```python
from build123d import *

# Parameters (mm, degrees)
F0_R     = 4.2534442679
F1_DEPTH = 20
F2_W     = 10.3906942531
F2_H     = 12.2660957277
F2_W_2   = 9.8304990679
F2_W_3   = 9.2522380874
F2_W_4   = 10.9689552337
F3_DEPTH = 10.16
F5_R     = 6.35
F6_DEPTH = 25.4
F7_R     = 6.35
F8_DEPTH = 25.4
F4_W     = 109.22
F4_H     = 58.420000254
F9_DEPTH = 12.7


# Not quite as in the source:
# - a feature names something its author has since deleted; it is built from what else it names


with BuildPart() as f1:
    # F0 (on Top) → F1 (new body)
    with BuildSketch(Plane.XY):
        Polygon((-67.5837442279, -21.374759078), (-67.5837442279, -75), (-7.2734476998, -75), (0, -75), (67.5837334, -75), (67.5837334, -21.374759078), (75, -21.374759078), (75, -5.6661395316), (75, 75), (-75, 75), (-75, -5.6661395316), (-75, -21.374759078), align=None)
        with BuildLine():
            ThreePointArc((-190.7009859405, 27.2364963511), (-152.5558792144, -43.9704630954), (-75, -21.374759078))
            Line((-75, -21.374759078), (-75, -5.6661395316))
            ThreePointArc((-75, -5.6661395316), (-127.811049195, -18.8460311242), (-161.148882109, 24.1807669913))
            ThreePointArc((-161.148882109, 24.1807669913), (-155.1100282823, 33.0940415029), (-154.4303864618, 43.8389149342))
            Line((-154.4303864618, 43.8389149342), (-140.2046696458, 49.3057770206))
            ThreePointArc((-140.2046696458, 49.3057770206), (-136.7560169722, 57.9771637157), (-145.6751462177, 60.7222112528))
            Line((-145.6751462177, 60.7222112528), (-146.0841166448, 60.4629836272))
            Line((-146.0841166448, 60.4629836272), (-158.5471573729, 52.5632328352))
            ThreePointArc((-158.5471573729, 52.5632328352), (-161.385975302, 55.4455313061), (-164.7362764103, 57.7131322838))
            Line((-164.7362764103, 57.7131322838), (-155.482622785, 75.8038009996))
            ThreePointArc((-155.482622785, 75.8038009996), (-159.2281719938, 84.7522052149), (-167.4260348338, 79.5658652979))
            Line((-167.4260348338, 79.5658652979), (-173.4289959882, 60.1528063587))
            ThreePointArc((-173.4289959882, 60.1528063587), (-174.9118696964, 60.1750253912), (-176.3924593558, 60.0898057902))
            Line((-176.3924593558, 60.0898057902), (-186.9047044679, 80.3893698915))
            ThreePointArc((-186.9047044679, 80.3893698915), (-195.4793934942, 84.7270210192), (-198.5276463049, 75.6139170472))
            Line((-198.5276463049, 75.6139170472), (-187.1383609375, 55.7931254681))
            ThreePointArc((-187.1383609375, 55.7931254681), (-189.6692112484, 53.4271036789), (-191.7647204388, 50.6680995766))
            Line((-191.7647204388, 50.6680995766), (-210.142074272, 59.3384667019))
            ThreePointArc((-210.142074272, 59.3384667019), (-220.775202398, 56.5846111171), (-213.1234756292, 48.7043692565))
            Line((-213.1234756292, 48.7043692565), (-194.9065059539, 38.4823538939))
            ThreePointArc((-194.9065059539, 38.4823538939), (-193.6469430671, 32.5441016935), (-190.7009859405, 27.2364963511))
        make_face()
        with BuildLine():
            Line((75, -5.6661395316), (75, -21.374759078))
            ThreePointArc((75, -21.374759078), (152.5558792144, -43.9704630954), (190.7009859405, 27.2364963511))
            ThreePointArc((190.7009859405, 27.2364963511), (193.6469430671, 32.5441016935), (194.9065059539, 38.4823538939))
            Line((194.9065059539, 38.4823538939), (213.1234756292, 48.7043692565))
            ThreePointArc((213.1234756292, 48.7043692565), (220.775202398, 56.5846111171), (210.142074272, 59.3384667019))
            Line((210.142074272, 59.3384667019), (191.7647204388, 50.6680995766))
            ThreePointArc((191.7647204388, 50.6680995766), (189.6692112484, 53.4271036789), (187.1383609375, 55.7931254681))
            Line((187.1383609375, 55.7931254681), (198.5276463049, 75.6139170472))
            ThreePointArc((198.5276463049, 75.6139170472), (195.4793934942, 84.7270210192), (186.9047044679, 80.3893698915))
            Line((186.9047044679, 80.3893698915), (176.3924593558, 60.0898057902))
            ThreePointArc((176.3924593558, 60.0898057902), (174.9118696964, 60.1750253912), (173.4289959882, 60.1528063587))
            Line((173.4289959882, 60.1528063587), (167.4260348338, 79.5658652979))
            ThreePointArc((167.4260348338, 79.5658652979), (159.2281719938, 84.7522052149), (155.482622785, 75.8038009996))
            Line((155.482622785, 75.8038009996), (164.7362764103, 57.7131322838))
            ThreePointArc((164.7362764103, 57.7131322838), (161.385975302, 55.4455313061), (158.5471573729, 52.5632328352))
            Line((158.5471573729, 52.5632328352), (146.0841166448, 60.4629836272))
            Line((146.0841166448, 60.4629836272), (145.6751462177, 60.7222112528))
            ThreePointArc((145.6751462177, 60.7222112528), (136.7560169722, 57.9771637157), (140.2046696458, 49.3057770206))
            Line((140.2046696458, 49.3057770206), (154.4303864618, 43.8389149342))
            ThreePointArc((154.4303864618, 43.8389149342), (155.1100282823, 33.0940415029), (161.148882109, 24.1807669913))
            ThreePointArc((161.148882109, 24.1807669913), (127.811049195, -18.8460311242), (75, -5.6661395316))
        make_face()
        with BuildLine():
            Line((0, -75), (-7.2734476998, -75))
            Line((-7.2734476998, -75), (-7.2734476998, -136.4104553148))
            ThreePointArc((-7.2734476998, -136.4104553148), (-3.6367238499, -136.120270713), (0, -136.4104553148))
            Line((0, -136.4104553148), (0, -75))
        make_face()
        with BuildLine():
            ThreePointArc((0, -136.4104553148), (-3.6367238499, -136.120270713), (-7.2734476998, -136.4104553148))
            ThreePointArc((-7.2734476998, -136.4104553148), (-18.5120008809, -176.508894443), (19.2968973343, -159.0538918972))
            ThreePointArc((19.2968973343, -159.0538918972), (13.8182786959, -144.1786148662), (0, -136.4104553148))
        make_face()
        with Locations((-3.6367238499, -159.0538918972)):
            Circle(F0_R, mode=Mode.SUBTRACT)
        with Locations((-3.6367238499, -159.0538918972)):
            Circle(F0_R)
    extrude(amount=F1_DEPTH)

    # F2 (on face) → F3 (join)
    with BuildSketch(Plane.XY.offset(20)):
        with Locations((-13.8693177141, -30.8799799532)):
            Rectangle(F2_W, F2_H)
        with Locations((-3.7587210536, -30.8799799532)):
            Rectangle(F2_W_2, F2_H)
        with Locations((5.782647524, -30.8799799532)):
            Rectangle(F2_W_3, F2_H)
        with Locations((15.8932441846, -30.8799799532)):
            Rectangle(F2_W_4, F2_H)
        with BuildLine():
            Line((-50.2273030579, -53.9529807866), (-61.5431257083, -48.187379539))
            ThreePointArc((-61.5431257083, -48.187379539), (-41.2897769448, -62.9757645575), (-55.8852143831, -42.5829306795))
            Line((-55.8852143831, -42.5829306795), (-50.2273030579, -53.9529807866))
        make_face()
        with BuildLine():
            Line((-14.4444061443, -55.5018670857), (-14.4444061443, -42.8018670857))
            ThreePointArc((-14.4444061443, -42.8018670857), (-18.5320544995, -67.5260564939), (-6.7041450331, -45.4331850503))
            Line((-6.7041450331, -45.4331850503), (-14.4444061443, -55.5018670857))
        make_face()
        with BuildLine():
            Line((19.0666168928, -56.657422334), (26.0705094181, -67.2515475689))
            ThreePointArc((26.0705094181, -67.2515475689), (15.4098006877, -44.4952804485), (19.0666168928, -69.357422334))
            Line((19.0666168928, -69.357422334), (19.0666168928, -56.657422334))
        make_face()
        with BuildLine():
            Line((51.4220893383, -56.0796447098), (64.1220893383, -56.0796447098))
            ThreePointArc((64.1220893383, -56.0796447098), (39.2223619287, -52.550246584), (62.1604119949, -62.8603840886))
            Line((62.1604119949, -62.8603840886), (51.4220893383, -56.0796447098))
        make_face()
    extrude(amount=F3_DEPTH)

    # F5 (on face) → F6 (cut)
    with BuildSketch(Plane.XY.offset(20)):
        with Locations((-3.6367238499, -159.0538918972)):
            Circle(F5_R)
    extrude(amount=-F6_DEPTH, mode=Mode.SUBTRACT)

    # F7 (on face) → F8 (cut)
    with BuildSketch(Plane.XY.offset(20)):
        with Locations((66.185079515, 67.0784339309)):
            Circle(F7_R)
    extrude(amount=-F8_DEPTH, mode=Mode.SUBTRACT)

    # F4 (on face) → F9 (join)
    with BuildSketch(Plane.XY.offset(20)):
        with Locations((-2.614335165, 37.8684338039)):
            Rectangle(F4_W, F4_H)
    extrude(amount=F9_DEPTH)


solid = f1.part
```
The model under review builds one solid part; all positions refer to its coordinate system, in mm. A direction names the side the tool comes from. Give positions to 0.01 mm unless a question says otherwise; leave off trailing zeros. Write each loop counter-clockwise with the first axis right and the second up, starting at its lowest first coordinate (ties: lowest second). Pieces come first, ordered by that corner, then holes.
(1) The part is to be moulded in two halves that separate along X. For faces 5 (the flat face through (21.378, -31, 25)), 6 (the flat face through (160.04, 66.89, 9.86)), 7 (the flat face through (-3, 8.658, 26)), say which applies: released by +X, released by -X, zero draft, split by the parting line, or undercut.
(2) Consider section C-C, the plane z = 10.5. Give the number of separate pieces and of enclosed holes in the cut face, and give its area (3 significant figures).
(3) Consider section B-B, the plane y = -131. Give the boundary of the cut face in (x, z), and give its area (3 significant figures).
(4) For P1, Ø8, axis at x = -70.5, z = 6.5, coming from the -Y side; P2, Ø2, axis at y = 31.5, z = 10.5, coming from the +X side; P3, Ø10, axis at y = 38.5, z = 7.5, coming from the +X side, all flat-tipped, find the tip position at first contact; note any pin that passes through.
(5) Tool access review of faces 1 (the cylindrical face through (155.06, 33.24, 9.86)), 2 (the flat face through (-15, -55, 30.16)), 3 (the flat face through (-1, -8, 0)), 4 (the flat face through (1, 75, 10)): name each direction out of +Z, -Z, +X, -X, +Y, -Y from which nothing blocks a thin tool from reaching the whole face with its end or side.
(6) Consider section A-A, the plane y = -11. Give the boundary of the cut face in (x, z).
(7) Consider section D-D, the plane x = -96. Give the boundary of the cut face in (y, z), and give its area (3 significant figures).
(8) To check wall thickness, follow L1, parallel to X at y = -13.5, z = 19.5; L2, parallel to X at y = 21, z = 11; L3, parallel to X at y = -111, z = 13. State the ranges of each line that lie inside material, in increasing order.
Returned:
1. face 5: released by +X
1. face 6: undercut
1. face 7: zero draft
2. separate pieces: 1
2. enclosed holes: 2
2. area: 36,400 mm2
3. outline: (-7.27, 0) - (0, 0) - (0, 20) - (-7.27, 20) - close
3. area: 145 mm2
4. P1: stops at y = -75
4. P2: stops at x = 193.63
4. P3: stops at x = 203.85
5. face 1: +Z, -Z
5. face 2: +Z, +X, -X, -Y
5. face 3: -Z, +X, -X, +Y, -Y
5. face 4: +Z, -Z, +Y
6. outline: (-186.27, 0) - (-142.21, 0) - (-142.21, 20) - (-186.27, 20) - close; (-80.8, 0) - (80.8, 0) - (80.8, 20) - (-80.8, 20) - close; (142.21, 0) - (186.27, 0) - (186.27, 20) - (142.21, 20) - close
7. outline: (-40.59, 0) - (-19.12, 0) - (-19.12, 20) - (-40.59, 20) - close
7. area: 429 mm2
8. L1: x = -185.09 to -138.72, -84.29 to 84.29, 138.72 to 185.09
8. L2: x = -191.58 to -160.79, -75 to 75, 160.79 to 191.58
8. L3: x = -7.27 to 0
